The listing builds one solid part. Answer for the finished solid, in the listing's coordinates (mm). Coordinates: 2 decimals unless noted, no trailing zeros. Loops run counter-clockwise (first coordinate to the right, second up) from the corner with the lowest first, then second, coordinate; pieces in that order, holes last. Notation, with made-up numbers: (63, 44) - (71, 44) arc R13 ccw to (71, 55) - close; hole circle Ø5 at (-2.75, 75.5). An arc over 180 degrees is marked (long way). Write each question's results on one line, items separated by ' | '. Start each with the question number.
(1) Find section D-D on x = 7. Determine the outline of the cut face in (y, z).
(2) Given pin 1 Ø12 at (x, z) = (-18, 10) entering from +Y; pin 2 Ø10 at (x, z) = (-4, 13) entering from +Y; pin 3 Ø12 at (y, z) = (-9.5, 23.5) entering from +X, each flat-ended and moving along its own axis, determine where each tip first touches the part or whether it passes through.
(3) Consider line 1 (Y direction, x = 0, z = 17); line 2 (Y direction, x = -1.5, z = 11); line 3 (Y direction, x = -8, z = 14.75). Determine where each line is inside the solid, lowest interval first. Write a range as from..to.
(4) Find section B-B on z = 14. Determine the outline of the cut face in (x, y).
(5) Determine the mould class of faces 1 (the flat face through (-7.49, -23.645, 12.818)), 2 (the flat face through (0, 0, 0)), 3 (the cylindrical face through (22.5, -0.3, 12.8)), 4 (the cylindrical face through (-0.228, -23.965, 12.818)) for opening direction X: released by +X, released by -X, zero draft, split by the parting line, or undercut.
(6) Find section C-C on y = 20.5. Determine the outline of the cut face in (x, z).
(7) Find section A-A on y = -25. Determine the outline of the cut face in (x, z), then the cut area to 3 significant figures.
from build123d import *

# Parameters (mm, degrees)
SKETCH_R  = 1.75
PAD_DEPTH = 26


with BuildPart() as part:
    # Sketch → Pad (new body)
    with BuildSketch(Plane.XY):
        with BuildLine():
            Line((0, 30.499996), (-15.190274, 16.598361))
            ThreePointArc((-15.190274, 16.598361), (-22.5, 0.001507), (-15.192497, -16.596326))
            Line((0, -30.500004), (-15.192497, -16.596326))
            Line((0, -30.500004), (15.190268, -16.598366))
            ThreePointArc((15.190268, -16.598366), (22.5, -3e-06), (15.190272, 16.598363))
            Line((0, 30.499996), (15.190272, 16.598363))
        make_face()
        with Locations((0, 25.7)):
            Circle(SKETCH_R, mode=Mode.SUBTRACT)
        with Locations((0, -25.7)):
            Circle(SKETCH_R, mode=Mode.SUBTRACT)
    extrude(amount=PAD_DEPTH)


solid = part.part
Values:
1) outline: (-24.09, 0) - (24.09, 0) - (24.09, 26) - (-24.09, 26) - close
2) pin 1: stops at y = 19.52 | pin 2: stops at y = 30.5 | pin 3: stops at x = 22.23
3) line 1: y = -30.5..-27.45, -23.95..23.95, 27.45..30.5 | line 2: y = -29.13..-26.6, -24.8..24.8, 26.6..29.13 | line 3: y = -23.18..23.18
4) outline: (-15.19, -16.6) - (0, -30.5) - (15.19, -16.6) arc R22.5 ccw to (15.19, 16.6) - (0, 30.5) - (-15.19, 16.6) arc R22.5 ccw to start; hole circle Ø3.5 at (0, -25.7); hole circle Ø3.5 at (0, 25.7)
5) face 1: released by -X | face 2: zero draft | face 3: released by +X | face 4: undercut
6) outline: (-10.93, 0) - (10.93, 0) - (10.93, 26) - (-10.93, 26) - close
7) outline: (-6.01, 0) - (-1.6, 0) - (-1.6, 26) - (-6.01, 26) - close; (1.6, 0) - (6.01, 0) - (6.01, 26) - (1.6, 26) - close | area: 229 mm²
